Geometry: final body of the model. Coordinates: model frame, mm. A direction names the side the tool comes from. Round coordinates to 2 decimals unless told otherwise and drop trailing zeros. Order: outer loops, then holes, each group sorted by start corner. A loop starts at its lowest first (then second) coordinate and runs counter-clockwise, first axis right, second up. Notation, with made-up numbers: M 20.5,-2 L 24.5,-2 A16 ccw 24.5,8 Z; hole C 31,59.25 d2. An arc over 180 degrees is marked long. Return JSON: item names as keys, results as strings. Group by question number.
Q1. Cut plane D-D on z = 11.75. Output: boundary loops of the cut face in (x, y), and give its area (3 significant figures).
Q2. Cut plane B-B on z = 6.35. Output: boundary loops of the cut face in (x, y), and give its area (3 significant figures).
Q3. Cut plane C-C on x = 0. Output: boundary loops of the cut face in (y, z).
Q4. Contact query for flat-ended pins moving along their axis: pin 1 (20.5 mm diameter, centred on x = 0, y = 0, fed in from -Z); pin 2 (1.5 mm diameter, centred on y = -15, z = 10.5, fed in from +X); pin 3 (3 mm diameter, centred on x = -30, y = 3, fed in from +Z). Output: stop coordinate, or through.
Q5. Mould query, pull axis X, two halves, no side actions, for faces 1 (the face through (6.35, 18, 10)), 2 (the face through (32, 0, 12.7)), 3 (the face through (-35.861, 0, 6)), 4 (the face through (17, 0, 10.16)). Classes: released by +X, released by -X, zero draft, split by the parting line, or undercut.
Q6. Ray query, probe 1 along X at (y, z) = (0, 7.5); probe 2 along X at (y, z) = (20.5, 9); probe 3 along Y at (x, z) = (0, 5.75). Return the intervals inside material, ascending.
Q7. Access query for faces 5 (the face through (-17, 0, 12.7)), 6 (the face through (-26.971, 0, 10)). Directions: +Z, -Z, +X, -X, +Y, -Y. A direction counts if a zero-diameter tool reaches every point of the face in a straight line with its end or side. Return the directions, or none.
Q8. Cut plane A-A on y = 0. Output: boundary loops of the cut face in (x, z).
```python
from build123d import *

# Parameters (mm, degrees)
F0_W     = 76.2
F0_H     = 50.8
F0_R     = 12.7
F1_DEPTH = 12.7
F2_W     = 6.35
F2_H     = 50.8
F3_DEPTH = 5.08
F5_DEPTH = 50.801
F6_R     = 2.2225
F7_DEPTH = 12.7


with BuildPart() as f1:
    # F0 (on Top) → F1 (new body)
    with BuildSketch(Plane.XY):
        with Locations((2.2386768513, 0)):
            Rectangle(F0_W, F0_H)
        Circle(F0_R, mode=Mode.SUBTRACT)
    extrude(amount=F1_DEPTH)

    # F2 (on face) → F3 (cut)
    with BuildSketch(Plane.XY.offset(12.7)):
        with Locations((-30.1463231487, 0)):
            Rectangle(F2_W, F2_H)
        with BuildLine():
            Line((-6.35, -10.9985226281), (-6.35, -25.4))
            Line((-6.35, -25.4), (6.35, -25.4))
            Line((6.35, -25.4), (6.35, -10.9985226281))
            ThreePointArc((6.35, -10.9985226281), (0, -12.7), (-6.35, -10.9985226281))
        make_face()
        with BuildLine():
            Line((6.35, 25.4), (-6.35, 25.4))
            Line((-6.35, 25.4), (-6.35, 10.9985226281))
            ThreePointArc((-6.35, 10.9985226281), (0, 12.7), (6.35, 10.9985226281))
            Line((6.35, 10.9985226281), (6.35, 25.4))
        make_face()
    extrude(amount=-F3_DEPTH, mode=Mode.SUBTRACT)

    # F4 (on face) → F5 (cut, through all)
    with BuildSketch(Plane.XZ.offset(25.4)):
        Polygon((23.3443384257, 12.7), (10.6443384257, 12.7), (9.1778687419, 10.16), (24.8108081094, 10.16), align=None)
    extrude(amount=-F5_DEPTH, mode=Mode.SUBTRACT)

    # F6 (on face) → F7 (join)
    with BuildSketch(Plane.YZ.offset(40.3386768513)):
        with Locations((0, 6.35)):
            Circle(F6_R)
    extrude(amount=F7_DEPTH)


solid = f1.part
```
Result sheet:
{
 "1": {"outline": "M -35.86,-25.4 L -33.32,-25.4 L -33.32,25.4 L -35.86,25.4 Z; M -26.97,-25.4 L -6.35,-25.4 L -6.35,-11 A12.7 cw -6.35,11 L -6.35,25.4 L -26.97,25.4 Z; M 6.35,-25.4 L 10.1,-25.4 L 10.1,-7.7 A12.7 cw 6.35,-11 Z; M 6.35,11 A12.7 cw 10.1,7.7 L 10.1,25.4 L 6.35,25.4 Z; M 23.89,-25.4 L 40.34,-25.4 L 40.34,25.4 L 23.89,25.4 Z", "area": "2,030 mm²"},
 "2": {"outline": "M -35.86,-25.4 L 40.34,-25.4 L 40.34,-2.22 L 53.04,-2.22 L 53.04,2.22 L 40.34,2.22 L 40.34,25.4 L -35.86,25.4 Z; hole C 0,0 d25.4", "area": "3,420 mm²"},
 "3": {"outline": "M -25.4,0 L -12.7,0 L -12.7,7.62 L -25.4,7.62 Z; M 12.7,0 L 25.4,0 L 25.4,7.62 L 12.7,7.62 Z"},
 "4": {"pin 1": "passes through", "pin 2": "stops at x = 40.34", "pin 3": "stops at z = 7.62"},
 "5": {"face 1": "undercut", "face 2": "zero draft", "face 3": "released by -X", "face 4": "undercut"},
 "6": {"probe 1": "x = -35.86 to -12.7, 12.7 to 53.04", "probe 2": "x = -35.86 to -33.32, -26.97 to -6.35, 6.35 to 40.34", "probe 3": "y = -25.4 to -12.7, 12.7 to 25.4"},
 "7": {"face 5": "+Z, +X, -X, +Y, -Y", "face 6": "+Z, +Y, -Y"},
 "8": {"outline": "M -35.86,0 L -12.7,0 L -12.7,12.7 L -26.97,12.7 L -26.97,7.62 L -33.32,7.62 L -33.32,12.7 L -35.86,12.7 Z; M 12.7,0 L 40.34,0 L 40.34,4.13 L 53.04,4.13 L 53.04,8.57 L 40.34,8.57 L 40.34,12.7 L 23.34,12.7 L 24.81,10.16 L 12.7,10.16 Z"}
}
